Could you check a few things on this model? Use its own coordinates, in mm. A direction names the side the tool comes from. Give positions to 0.01 mm unless a question says otherwise; leave off trailing zeros. Order: outer loops, then holes, each group sorted by start corner. A loop starts at its lowest first (then second) coordinate and runs counter-clockwise, first axis right, second up. Notation, with made-up numbers: (86, 5.5) - (124, 5.5) arc R9 ccw to (124, 19.5) - close; hole circle Ø4 at (89, 78). An arc over 180 degrees is marked (long way). Put each result on its own line as item: value.
from build123d import *

# Parameters (mm, degrees)
ESQUISSE2_R                  = 8.5
BOSS_EXTRU_1_DEPTH           = 23
ENL_V_START                  = 23
ESQUISSE3_R                  = 2
ENL_V_MAT_EXTRU_3_DEPTH      = 24
ENL_V_MAT_EXTRU_3_DEPTH_BACK = 8
ENL_V_START_2                = -12
ESQUISSE4_R                  = 1.5
ENL_V_MAT_EXTRU_4_DEPTH      = 8
BOSS_EXTRU_2_DEPTH           = 28
CONG_5_R                     = 1.8
ENL_V_MAT_EXTRU_5_DEPTH      = 5
ESQUISSE7_R                  = 1.5
ESQUISSE7_W                  = 1.9
ESQUISSE7_H                  = 0.1
ENL_V_MAT_EXTRU_6_DEPTH      = 3
CONG_6_R                     = 3


with BuildPart() as part:
    # Esquisse2 → Boss.-Extru.1 (new body)
    with BuildSketch(Plane(origin=(0, 0, 0), x_dir=(1, 0, 0), z_dir=(0, 1, 0))):
        Polygon((15, 12), (-15, 12), (-17.892304845, 6.990381057), (-2.892304845, -18.990381057), (2.892304845, -18.990381057), (17.892304845, 6.990381057), align=None)
        Circle(ESQUISSE2_R, mode=Mode.SUBTRACT)
    extrude(amount=BOSS_EXTRU_1_DEPTH)

    # Esquisse3 → Enlèv. mat.-Extru.3 (cut, two sides)
    with BuildSketch(Plane(origin=(0, 0, 0), x_dir=(1, 0, 0), z_dir=(0, 1, 0)).offset(ENL_V_START)) as enl_v_mat_extru_3_sk:
        with Locations((-12.982050808, 7.495190528)):
            Circle(ESQUISSE3_R)
        with Locations((12.982050808, 7.495190528)):
            Circle(ESQUISSE3_R)
        with Locations((0, -14.990381057)):
            Circle(ESQUISSE3_R)
    extrude(amount=ENL_V_MAT_EXTRU_3_DEPTH, mode=Mode.SUBTRACT)
    extrude(enl_v_mat_extru_3_sk.sketch, amount=-ENL_V_MAT_EXTRU_3_DEPTH_BACK, mode=Mode.SUBTRACT)

    # Esquisse4 → Enlèv. mat.-Extru.4 (cut)
    with BuildSketch(Plane.XY.offset(ENL_V_START_2)):
        with Locations((-11, 11)):
            Circle(ESQUISSE4_R)
        with Locations((11, 11)):
            Circle(ESQUISSE4_R)
        with Locations((11, 3)):
            Circle(ESQUISSE4_R)
        with Locations((-11, 3)):
            Circle(ESQUISSE4_R)
    extrude(amount=ENL_V_MAT_EXTRU_4_DEPTH, mode=Mode.SUBTRACT)

    # Esquisse5 → Boss.-Extru.2 (add)
    with BuildSketch(Plane(origin=(0, 0, 0), x_dir=(1, 0, 0), z_dir=(0, 1, 0))):
        with BuildLine():
            Line((13.220508076, -17.101408311), (15.370508076, -13.377499075))
            ThreePointArc((15.370508076, -13.377499075), (15.510368667, -12.315152412), (14.85807251, -11.465063509))
            Line((14.85807251, -11.465063509), (14.68486743, -11.365063509))
            ThreePointArc((14.68486743, -11.365063509), (14.032571273, -10.514974607), (14.172431864, -9.452627944))
            Line((14.172431864, -9.452627944), (15.272431864, -7.547372056))
            ThreePointArc((15.272431864, -7.547372056), (16.122520766, -6.895075899), (17.18486743, -7.034936491))
            Line((17.18486743, -7.034936491), (17.35807251, -7.134936491))
            ThreePointArc((17.35807251, -7.134936491), (18.420419174, -7.274797082), (19.270508076, -6.622500925))
            Line((19.270508076, -6.622500925), (21.420508076, -2.898591689))
            ThreePointArc((21.420508076, -2.898591689), (21.600328836, -1.532717408), (20.761662349, -0.439745962))
            Line((20.761662349, -0.439745962), (20.415252187, -0.239745962))
            ThreePointArc((20.415252187, -0.239745962), (19.049377906, -0.059925202), (17.956406461, -0.898591689))
            Line((17.956406461, -0.898591689), (17.756406461, -1.24500185))
            ThreePointArc((17.756406461, -1.24500185), (16.663435015, -2.083668338), (15.297560734, -1.903847577))
            Line((15.297560734, -1.903847577), (13.392304845, -0.803847577))
            Line((13.392304845, -0.803847577), (7.392304845, -11.196152423))
            Line((7.392304845, -11.196152423), (9.297560734, -12.296152423))
            ThreePointArc((9.297560734, -12.296152423), (10.136227221, -13.389123868), (9.956406461, -14.75499815))
            Line((9.956406461, -14.75499815), (9.756406461, -15.101408311))
            ThreePointArc((9.756406461, -15.101408311), (9.5765857, -16.467282592), (10.415252187, -17.560254038))
            Line((10.415252187, -17.560254038), (10.761662349, -17.760254038))
            ThreePointArc((10.761662349, -17.760254038), (12.12753663, -17.940074798), (13.220508076, -17.101408311))
        make_face()
        with BuildLine():
            Line((-19.270508076, -6.622500925), (-21.420508076, -2.898591689))
            ThreePointArc((-21.420508076, -2.898591689), (-21.600328836, -1.532717408), (-20.761662349, -0.439745962))
            Line((-20.761662349, -0.439745962), (-20.415252187, -0.239745962))
            ThreePointArc((-20.415252187, -0.239745962), (-19.049377906, -0.059925202), (-17.956406461, -0.898591689))
            Line((-17.956406461, -0.898591689), (-17.756406461, -1.24500185))
            ThreePointArc((-17.756406461, -1.24500185), (-16.663435015, -2.083668338), (-15.297560734, -1.903847577))
            Line((-15.297560734, -1.903847577), (-13.392304845, -0.803847577))
            Line((-13.392304845, -0.803847577), (-7.392304845, -11.196152423))
            Line((-7.392304845, -11.196152423), (-9.297560734, -12.296152423))
            ThreePointArc((-9.297560734, -12.296152423), (-10.136227221, -13.389123868), (-9.956406461, -14.75499815))
            Line((-9.956406461, -14.75499815), (-9.756406461, -15.101408311))
            ThreePointArc((-9.756406461, -15.101408311), (-9.5765857, -16.467282592), (-10.415252187, -17.560254038))
            Line((-10.415252187, -17.560254038), (-10.761662349, -17.760254038))
            ThreePointArc((-10.761662349, -17.760254038), (-12.12753663, -17.940074798), (-13.220508076, -17.101408311))
            Line((-13.220508076, -17.101408311), (-15.370508076, -13.377499075))
            ThreePointArc((-15.370508076, -13.377499075), (-15.510368667, -12.315152412), (-14.85807251, -11.465063509))
            Line((-14.85807251, -11.465063509), (-14.68486743, -11.365063509))
            ThreePointArc((-14.68486743, -11.365063509), (-14.032571273, -10.514974607), (-14.172431864, -9.452627944))
            Line((-14.172431864, -9.452627944), (-15.272431864, -7.547372056))
            ThreePointArc((-15.272431864, -7.547372056), (-16.122520766, -6.895075899), (-17.18486743, -7.034936491))
            Line((-17.18486743, -7.034936491), (-17.35807251, -7.134936491))
            ThreePointArc((-17.35807251, -7.134936491), (-18.420419174, -7.274797082), (-19.270508076, -6.622500925))
        make_face()
    extrude(amount=BOSS_EXTRU_2_DEPTH)

    # Congé5
    cong_5_edges = [part.edges().sort_by_distance(p)[0] for p in [
        (-7.392304845, 11.5, 11.196152423),
        (7.392304845, 11.5, 11.196152423),
        (13.392304845, 11.5, 0.803847577),
        (-13.392304845, 11.5, 0.803847577),
    ]]
    fillet(cong_5_edges, radius=CONG_5_R)

    # Esquisse6 → Enlèv. mat.-Extru.5 (cut)
    with BuildSketch(Plane(origin=(0, 0, 0), x_dir=(1, 0, 0), z_dir=(0, 1, 0)).offset(ENL_V_START)):
        Polygon((-13.392304845, -0.803847577), (-7.392304845, -11.196152423), (-7.478907386, -11.246152423), (-13.478907386, -0.853847577), align=None)
        Polygon((7.392304845, -11.196152423), (13.392304845, -0.803847577), (13.478907386, -0.853847577), (7.478907386, -11.246152423), align=None)
    extrude(amount=ENL_V_MAT_EXTRU_5_DEPTH, mode=Mode.SUBTRACT)

    # Esquisse7 → Enlèv. mat.-Extru.6 (cut)
    with BuildSketch(Plane(origin=(0, 0, -12), x_dir=(-1, 0, 0), z_dir=(0, 0, -1))):
        Polygon((15, 0), (0.85, 0), (-0.85, 0), (-15, 0), (-15, 14.1), (-15.1, 14.1), (-15.1, -0.1), (15.1, -0.1), (15.1, 14.1), (15, 14.1), align=None)
        Polygon((-0.85, 0), (0.85, 0), (15, 0), (15, 14.1), (0.95, 14.1), (0.95, 23), (-0.95, 23), (-0.95, 14.1), (-15, 14.1), (-15, 0), align=None)
        with Locations((-11, 3)):
            Circle(ESQUISSE7_R, mode=Mode.SUBTRACT)
        with Locations((-11, 11)):
            Circle(ESQUISSE7_R, mode=Mode.SUBTRACT)
        with Locations((11, 3)):
            Circle(ESQUISSE7_R, mode=Mode.SUBTRACT)
        with Locations((11, 11)):
            Circle(ESQUISSE7_R, mode=Mode.SUBTRACT)
        with Locations((0, 23.05)):
            Rectangle(ESQUISSE7_W, ESQUISSE7_H)
    extrude(amount=-ENL_V_MAT_EXTRU_6_DEPTH, mode=Mode.SUBTRACT)

    # Congé6
    cong_6_edges = [part.edges().sort_by_distance(p)[0] for p in [
        (-15.1, 14.1, -10.41339746),
        (15.1, 14.1, -10.41339746),
    ]]
    fillet(cong_6_edges, radius=CONG_6_R)


solid = part.part
1) Suppose I cut it at D-D, the plane x = -11.5. List the corners of the cut face in (y, z) for me.
Filled in:
outline: (0, -9) - (1.59, -9) - (1.59, -4) - (4.41, -4) - (4.41, -9) - (9.59, -9) - (9.59, -4) - (12.41, -4) - (12.41, -9) - (14.1, -9) - (14.1, -12) - (23, -12) - (23, -8.84) - (15, -8.84) - (15, -6.15) - (23, -6.15) - (23, 4.28) - (28, 4.28) - (28, 17.99) - (0, 17.99) - close
2) If I drill on line 1 (Y direction, x = 11, z = -6); line 2 (X direction, y = 21, z = 15); line 3 (Z direction, x = -14.5, y = 16.75), over which ranges is the centre line in solid material (lowest first)? Write a range as [from, to].
Filled in:
line 1: y = [0, 1.5], [4.5, 9.5], [12.5, 23]
line 2: x = [-14.43, -9.81], [-5.2, -2], [2, 5.2], [9.81, 14.43]
line 3: z = [-12, -8.8], [-6.19, -1.11], [1.33, 8.89], [11.24, 14.89]
3) Suppose I cut it at A-A, the plane x = 0. List the corners of the cut face in (y, z) for me, and give its area (3 significant figures).
Filled in:
outline: (0, -9) - (23, -9) - (23, -8.5) - (0, -8.5) - close; (0, 8.5) - (23, 8.5) - (23, 12.99) - (15, 12.99) - (15, 16.99) - (23, 16.99) - (23, 18.99) - (0, 18.99) - close
area: 221 mm^2
4) Suppose I cut it at B-B, the plane z = -4.5. List the corners of the cut face in (x, y) for me, and give its area (3 significant figures).
Filled in:
outline: (-16.45, 0) - (-7.21, 0) - (-7.21, 23) - (-16.45, 23) - close; (7.21, 0) - (16.45, 0) - (16.45, 23) - (7.21, 23) - close; hole circle Ø3 at (-11, 3); hole circle Ø3 at (-11, 11); hole circle Ø3 at (11, 3); hole circle Ø3 at (11, 11)
area: 397 mm^2
5) Which directions (+Z, -Z, +X, -X, +Y, -Y) give clear straight access to the entire face, cutting with the end or side of a thin tool? Please do faces 1 (the cylindrical face through (-14.2, 13.24, -10.48)), 2 (the flat face through (-4.718, 11.339, 15.829)), 3 (the cylindrical face through (-12.5, 11.07, -6.54)), 4 (the cylindrical face through (0.923, 19.056, 16.765)), 5 (the cylindrical face through (16.68, 13.8, 2.08)).
Filled in:
face 1: -Z, -Y
face 2: +Z, +Y, -Y
face 3: -Z
face 4: +Y
face 5: +Y, -Y
6) I'm going to push flat-ended pins straight in: pin 1 (5 mm diameter, centred on x = 11, y = 11, fed in from -Z); pin 2 (0.9 mm diameter, centred on y = 20.5, z = -11, fed in from -X); pin 3 (1 mm diameter, centred on x = 6, z = 12.5, fed in from +Y). Where does each tip first touch, or does it pass through?
Filled in:
pin 1: stops at z = -9
pin 2: stops at x = -15.84
pin 3: stops at y = 23
7) We'd pull the mould along Z, two halves only. Please class faces 6 (the cylindrical face through (-12.108, 13.804, 17.945)), 7 (the cylindrical face through (-15.514, 13.804, 12.33)), 8 (the flat face through (15.1, 6, -10)): pulls with the +Z half, pulls with the -Z half, needs draft (parallel to the pull), parting line crosses it, or undercut.
Filled in:
face 6: pulls with the +Z half
face 7: undercut
face 8: needs draft
8) Suppose I cut it at C-C, the plane z = 14. List the corners of the cut face in (x, y) for me, and give its area (3 significant figures).
Filled in:
outline: (-15.01, 0) - (-10.19, 0) - (-10.19, 28) - (-15.01, 28) - close; (-5.77, 0) - (5.77, 0) - (5.77, 23) - (1.74, 23) - (1.74, 15) - (-1.74, 15) - (-1.74, 23) - (-5.77, 23) - close; (10.19, 0) - (15.01, 0) - (15.01, 28) - (10.19, 28) - close
area: 508 mm^2
